Autodesk Inventor part; units mm, degrees
ref_plane "YZ Plane" through (0, 0, 0) normal (1, 0, 0) x (0, 1, 0)
ref_plane "XZ Plane" through (0, 0, 0) normal (0, 1, 0) x (-1, 0, 0)
ref_plane "XY Plane" through (0, 0, 0) normal (0, 0, 1) x (1, 0, 0)
sketch "スケッチ1" plane through (0, 0, 0) normal (0, 1, 0) x (-1, 0, 0)
  line L0 (15, 2.5) -> (-15, 2.5)
  line L1 (-15, 2.5) -> (-15, -2.5)
  line L2 (-15, -2.5) -> (15, -2.5)
  line L3 (15, -2.5) -> (15, 2.5)
  line L4 (15, 2.5) -> (-15, -2.5) construction
  line L5 (-15, 2.5) -> (15, -2.5) construction
  point P0 (0, 0)
  dimension "d0" = 30
  dimension "d1" = 5
extrude "押し出し1" add sketch "スケッチ1" along normal blind 7
sketch "スケッチ2" plane through (0, 7, 0) normal (0, 1, 0) x (1, 0, 0)
  circle A0 centre (0, 12.5) radius 2.9
  circle A1 centre (0, 12.5) radius 5.3852
  line L0 (-11, 10.5) -> (-5, 10.5)
  line L1 (-5, 10.5) -> (-5, 2.5)
  line L2 (15, 2.5) -> (-15, 2.5)
  line L3 (0, -8.1348) -> (0, 42.7212)
  line L4 (-15, -2.5) -> (15, -2.5)
  line L5 (15, -2.5) -> (15, 2.5)
  line L6 (15, 2.5) -> (-15, 2.5)
  line L7 (-15, 2.5) -> (-15, -2.5)
  line L8 (-15, -2.5) -> (15, -2.5)
  line L9 (-11, 10.5) -> (-11, 12)
  line L10 (-11, 12) -> (0, 12)
  line L11 (11, 10.5) -> (5, 10.5)
  line L12 (5, 10.5) -> (5, 2.5)
  line L13 (11, 10.5) -> (11, 12)
  line L14 (11, 12) -> (0, 12)
  point P0 (0, 0)
  point P1 (2.8566, 12)
  point P2 (-2.8566, 12)
  dimension "d5" = 5.8
  dimension "d9" = 6
  dimension "d10" = 10
  dimension "d40" = 0.5
  dimension "d41" = 15
  dimension "d42" = 1.5
extrude "押し出し2" add sketch "スケッチ2" along normal blind 6 contours L14 A1 L3 A0 | A0 L3 A1 L10 | L14 L13 L11 A1 | A1 L0 L9 L10 | L3 L2 L1 A1 | A1 L12 L2 L3 | L3 L4 L7 L2 | L2 L5 L4 L3 picked at (0.6464, 8.0199) picked at (-0.6464, 8.0199)
sketch "スケッチ4" plane through (0, 0, 0) normal (0, -1, 0) x (1, 0, 0)
  line L0 (-15, 2.5) -> (15, 2.5)
  line L1 (-15, -2.5) -> (-15, 2.5)
  line L2 (-15, 2.5) -> (15, 2.5)
  circle A0 centre (-12.5, 0) radius 1.6
  line L3 (0, 2.5) -> (0, -2.5)
  circle A1 centre (12.5, 0) radius 1.6
  point P0 (0, 0)
  point P1 (-15, 0)
  dimension "d78" = 3.2
  dimension "d79" = 2.5
extrude "押し出し4" cut sketch "スケッチ4" against normal blind 5
sketch "スケッチ5" plane through (-11, 7, -10.5) normal (0, 0, 1) x (1, 0, 0)
  circle A0 centre (3, 3) radius 1.1
  circle A1 centre (19, 3) radius 1.1
  line L0 (0, 6) -> (6, 6)
  line L1 (0, 0) -> (0, 6)
  line L2 (19, 5.3) -> (17, 4.1528)
  line L3 (17, 4.1528) -> (17, 1.8472)
  line L4 (17, 1.8472) -> (19, 0.7)
  line L5 (19, 0.7) -> (21, 1.8472)
  line L6 (21, 1.8472) -> (21, 4.1528)
  line L7 (21, 4.1528) -> (19, 5.3)
  line L8 (17, 1.8472) -> (21, 4.1528)
  line L9 (17, 4.1528) -> (21, 1.8472)
  line L10 (19, 5.3) -> (19, 0.7)
  line L11 (16.9, 4.2107) -> (19, 5.4153)
  line L12 (19, 5.4153) -> (21.1, 4.2107)
  line L13 (21.1, 4.2107) -> (21.1, 1.7893)
  line L14 (21.1, 1.7893) -> (19, 0.5847)
  line L15 (19, 0.5847) -> (16.9, 1.7893)
  line L16 (16.9, 1.7893) -> (16.9, 4.2107)
  line L17 (16, 6) -> (22, 6)
  line L18 (22, 0) -> (22, 6)
  point P0 (11, -7)
  point P1 (3, 6)
  point P2 (0, 3)
  point P3 (19, 6)
  point P4 (22, 3)
  dimension "d0" = 30
  dimension "d1" = 5
  dimension "d27" = 2.2
  dimension "d28" = 2.2
  dimension "d29" = 4.6
  dimension "d31" = 4
  dimension "d35" = 0.1
extrude "押し出し5" cut sketch "スケッチ5" against normal blind 0.75 contours A1 L9 L8 | A1 L8 L6 L9 | L8 L10 A1 | A1 L10 L7 L8 | L9 L5 L10 A1 | A1 L10 L9 | L10 L9 A1 | A1 L9 L2 L10 | L10 A1 L8 | L8 A1 L9 | L10 L4 L8 A1 | A1 L8 L3 L9 | L11 L12 L13 L14 L15 L16
extrude "押し出し6" cut sketch "スケッチ5" against normal through all contours A0
extrude "押し出し7" cut sketch "スケッチ5" against normal through all contours A1 L9 L8 | L8 L10 A1 | A1 L10 L9 | L10 L9 A1 | L10 A1 L8 | L8 A1 L9
sketch "スケッチ7" plane through (15, 0, -2.5) normal (0, 0, -1) x (-1, 0, 0)
  line L0 (10, 7.5) -> (0, 7.5)
  line L1 (0, 0) -> (0, 13)
  line L2 (10, 13) -> (10, 7.5)
  circle A0 centre (7, 10) radius 1.1
  line L3 (4, 7) -> (12.1434, 7)
  line L4 (12.1434, 7) -> (12.1434, 13)
  line L5 (4, 13) -> (12.1434, 13)
  line L6 (4, 7) -> (4, 13)
  line L7 (0, 0) -> (30, 0)
  line L8 (30, 0) -> (30, 13)
  line L9 (20, 13) -> (30, 13)
  line L10 (20, 7) -> (20, 13)
  line L11 (10, 7) -> (20, 7)
  line L12 (10, 7) -> (10, 13)
  line L13 (0, 13) -> (10, 13)
  line L14 (0, 0) -> (0, 13)
  line L15 (15, 13) -> (15, 0)
  line L16 (20, 7.5) -> (30, 7.5)
  line L17 (20, 13) -> (20, 7.5)
  dimension "d53" = 0.5
extrude "押し出し8" cut sketch "スケッチ7" against normal through all contours L0 L6 L5 L2 | L0 L1 L13 L6 | L10 L9 L8 L16 | A0
chamfer "面取り6" distance 3 angle 45 2 edges at (5, 7.5, 0) (-5, 7.5, 0)
chamfer "面取り7" distance 2 angle 45 2 edges at (15, 7.5, 0) (-15, 7.5, 0)
chamfer "面取り8" distance 2.5 angle 45 2 edges at (5, 13, -4) (-5, 13, -4)
chamfer "面取り9" distance 2 angle 45 11 edges at (-10.5, 7.5, 2.5) (-6.5, 9, 2.5) (0, 13, 2.5) (6.5, 9, 2.5) (10.5, 7.5, 2.5) (-14, 6.5, -2.5) (-10.5, 7.5, -2.5) (-6.5, 9, -2.5) (6.5, 9, -2.5) (10.5, 7.5, -2.5) (14, 6.5, -2.5)
sketch "スケッチ9" plane through (0, 13, 0) normal (0, 1, 0) x (1, 0, 0)
  circle A0 centre (0, 6) radius 1.25
  point P0 (0, 0)
  dimension "d74" = 2.5
  dimension "d75" = 6
extrude "押し出し9" cut sketch "スケッチ9" against normal through all
sketch "スケッチ10" plane through (0, 7, 0) normal (0, -1, 0) x (1, 0, 0)
  line L0 (5, -2.5) -> (5, -10.5)
  line L1 (5, -5) -> (3, -5)
  line L2 (3, -5) -> (0, -3.5)
  line L3 (0, -3.5) -> (-3, -5)
  line L4 (-3, -5) -> (-5, -5)
  line L5 (15, -2.5) -> (-15, -2.5)
  line L6 (-5, -10.5) -> (-5, -2.5)
  point P0 (0, 0)
  dimension "d80" = 2.5
  dimension "d81" = 1.5
  dimension "d82" = 2
split body "分割2" sketch "スケッチ10" result one side removed curves L1 L2 L3 L4 removed pieces at (2.3905, 1.8333, 2)
properties part number "mounter_top"
Build history of the part. All positions in model axes, mm. A direction names the side the tool comes from. Give positions to 0.01 mm unless a question says otherwise; leave off trailing zeros. Loops run counter-clockwise (first coordinate to the right, second up) from the corner with the lowest first, then second, coordinate; pieces in that order, holes last. Notation, with made-up numbers: (-36, 57) -> (21, 57) arc R23 ccw to (21, 96) -> close; hole circle Ø7 at (1, -40). An arc over 180 degrees is marked (long way). Answer in a Markdown table with one row per item.
Item 1: Slice it at B-B on y = 10. Write the cut outline in (x, z).
Findings below:
| item | result |
|---|---|
| outline | (-11, -12) -> (-9.1, -12) -> (-9.1, -10.5) -> (-11, -10.5) -> close; (-6.9, -12) -> (-2.86, -12) arc R2.9 cw to (2.86, -12) -> (6.9, -12) -> (6.9, -11.25) -> (5.9, -11.25) -> (5.9, -10.5) -> (5, -10.5) -> (5, -5) -> (3, -5) -> (0, -3.5) -> (-3, -5) -> (-5, -5) -> (-5, -10.5) -> (-6.9, -10.5) -> close; (9.1, -12) -> (11, -12) -> (11, -10.5) -> (10.1, -10.5) -> (10.1, -11.25) -> (9.1, -11.25) -> close; hole circle Ø2.5 at (0, -6) |
Item 2: Slice it at D-D on y = 7.9. Write the cut outline in (x, z).
Findings below:
| item | result |
|---|---|
| outline | (-11, -12) -> (-2.86, -12) arc R2.9 cw to (2.86, -12) -> (11, -12) -> (11, -10.5) -> (8.55, -10.5) -> (8.55, -11.25) -> (7.45, -11.25) -> (7.45, -10.5) -> (5, -10.5) -> (5, -5) -> (3, -5) -> (0, -3.5) -> (-3, -5) -> (-5, -5) -> (-5, -10.5) -> (-11, -10.5) -> close; hole circle Ø2.5 at (0, -6) |
Item 3: Mould opens along X. For faces 1 (the flat face through (-4, 9, -5)), 2 (the flat face through (-5, 9, -8)), 3 (the cylindrical face through (-0.27, 10.04, -4.78)) say: pulls with the +X half, pulls with the -X half, needs draft (parallel to the pull), parting line crosses it, or undercut.
Findings below:
| item | result |
|---|---|
| face 1 | needs draft |
| face 2 | pulls with the -X half |
| face 3 | undercut |
Item 4: Slice it at A-A on z = -6. Write the cut outline in (x, y), plus the area to 3 significant figures.
Findings below:
| item | result |
|---|---|
| outline | (-5, 7) -> (-1.25, 7) -> (-1.25, 13) -> (-2.5, 13) -> (-5, 10.5) -> close; (1.25, 7) -> (5, 7) -> (5, 10.5) -> (2.5, 13) -> (1.25, 13) -> close |
| area | 38.8 mm² |
Item 5: Flat gauge pins, fed straight in: P1, Ø3, axis at y = 9, z = -7.5, coming from the -X side; P2, Ø1.8, axis at x = 6.5, y = 10.5, coming from the +Z side; P3, Ø1.6, axis at x = -3.5, y = 10, coming from the +Z side; P4, Ø2, axis at x = -8, y = 10, coming from the -Z side. Where does each tip first touch, or does it go through?
Findings below:
| item | result |
|---|---|
| P1 | stops at x = -5 |
| P2 | stops at z = -10.5 |
| P3 | stops at z = -4.85 |
| P4 | passes through |
Item 6: Probe line 1 along Y through (x, z) = (-8, -11.5); line 2 along X through (y, z) = (8.55, -6); line 3 along X through (y, z) = (7.5, -7.5). List the from-to ranges inside material, lowest first. Write a range as [from, to].
Findings below:
| item | result |
|---|---|
| line 1 | y = [7, 8.9], [11.1, 13] |
| line 2 | x = [-5, -1.25], [1.25, 5] |
| line 3 | x = [-5, 5] |
Item 7: Tool access for faces 4 (the flat face through (-11, 10, -11)), 5 (the flat face through (6.8, 12, -10.5)), 6 (the flat face through (9.065, 8.195, -10.87)), 7 (the cylindrical face through (8.508, 9.024, -11.62)), 8 (the flat face through (-3.7, 11.8, -7.6)): list every direction of +Z, -Z, +X, -X, +Y, -Y with a clear straight run to the whole face (end or side of a thin tool).
Findings below:
| item | result |
|---|---|
| face 4 | +Z, -Z, -X, +Y, -Y |
| face 5 | +Z, +X, +Y |
| face 6 | +Z |
| face 7 | +Z, -Z |
| face 8 | +Z, -X, +Y |
Item 8: Slice it at C-C on x = -8. Write the cut outline in (y, z).
Findings below:
| item | result |
|---|---|
| outline | (7, -12) -> (8.9, -12) -> (8.9, -10.5) -> (7, -10.5) -> close; (11.1, -12) -> (13, -12) -> (13, -10.5) -> (11.1, -10.5) -> close |
